Build history of the part. All positions in model axes, mm. A direction names the side the tool comes from. Give positions to 0.01 mm unless a question says otherwise; leave off trailing zeros. Loops run counter-clockwise (first coordinate to the right, second up) from the corner with the lowest first, then second, coordinate; pieces in that order, holes last. Notation, with made-up numbers: M -23,57.25 L 19,57.25 A24 cw 19,93.25 Z; hole C -29,74 d6. An arc over 180 degrees is marked long. Answer as a JSON object with one key per item and string values. Group by question number.
1. 3-axis set-ups, long thin cutter, end or side, ignore diameter. For faces 4 (the face through (18.298, -103, -40)), 5 (the face through (16.898, -103, -43)): which of +Z, -Z, +X, -X, +Y, -Y reach the whole face in a straight line?
2. Slice it at C-C (z = -36.75). List the corners of the cut face in (x, y).
3. Mould opens along Y. For faces 1 (the face through (21.729, -101.846, -48.98)), 2 (the face through (26.698, -103, -48)), 3 (the face through (21, -107.117, -47)) say: released by +Y, released by -Y, zero draft, split by the parting line, or undercut.
4. Slice it at D-D (z = -42). List the corners of the cut face in (x, y), then the cut area to 3 significant figures.
5. Drill centre lines: line 1 along Z through (x, y) = (22.5, -104.75); line 2 along Y through (x, z) = (19.75, -48.5); line 3 along Y through (x, z) = (22, -48.25). Where is each one in solid material? Low to high. Write a range as [from, to].
6. Drop flat-ended pins along their axis: pin 1 Ø1 at (x, y) = (21, -100.5) entering from +Z; pin 2 Ø3 at (y, z) = (-103.5, -36.5) entering from +X; pin 3 Ø1.4 at (y, z) = (-101.36, -48.34) entering from -X. Give the stop position or say it passes through.
7. Slice it at A-A (y = -101). List the corners of the cut face in (x, z), then the cut area to 3 significant figures.
8. Slice it at B-B (x = 26). List the corners of the cut face in (y, z).
from build123d import *

# Parameters (mm, degrees)
CROQUIS1_W                = 6
CROQUIS1_H                = 7.864261992
SALIENTE_EXTRUIR1_DEPTH   = 9.8
CROQUIS2_W                = 1.4
CROQUIS2_H                = 7.864261992
SALIENTE_EXTRUIR2_DEPTH   = 11.5
CROQUIS3_R                = 1
CORTAR_EXTRUIR1_DEPTH     = 1.4
TALADRO_ROSCADO_M21_D     = 1.6
TALADRO_ROSCADO_M21_DEPTH = 13
TALADRO_ROSCADO_M21_TIP   = 0.480688495


with BuildPart() as part:
    # Croquis1 → Saliente-Extruir1 (new body)
    with BuildSketch(Plane.ZY.offset(-26.697955236)):
        with Locations((-48.344788292, -103.185244075)):
            Rectangle(CROQUIS1_W, CROQUIS1_H)
    extrude(amount=SALIENTE_EXTRUIR1_DEPTH)

    # Croquis2 → Saliente-Extruir2 (add)
    with BuildSketch(Plane.XY.offset(-45.344788292)):
        with Locations((17.597955236, -103.185244075)):
            Rectangle(CROQUIS2_W, CROQUIS2_H)
    extrude(amount=SALIENTE_EXTRUIR2_DEPTH)

    # Croquis3 → Cortar-Extruir1 (cut)
    with BuildSketch(Plane(origin=(18.297955236, 0, 0), x_dir=(0, 0, -1), z_dir=(1, 0, 0))):
        with Locations((36.344788292, -103.185244075)):
            Circle(CROQUIS3_R)
    extrude(amount=-CORTAR_EXTRUIR1_DEPTH, mode=Mode.SUBTRACT)

    # Taladro roscado M21
    with Locations(Plane(origin=(26.697955236, 0, 0), x_dir=(0, 0, -1), z_dir=(1, 0, 0))):
        with Locations((48.344788292, -104.677829932), (48.344788292, -101.359309211)):
            Hole(TALADRO_ROSCADO_M21_D / 2, depth=TALADRO_ROSCADO_M21_DEPTH)
            with Locations((0, 0, -(TALADRO_ROSCADO_M21_DEPTH + TALADRO_ROSCADO_M21_TIP / 2))):  # 118° drill point
                Cone(0, TALADRO_ROSCADO_M21_D / 2, TALADRO_ROSCADO_M21_TIP, mode=Mode.SUBTRACT)


solid = part.part
Established:
{
 "1": {"face 4": "+Z, +X, +Y, -Y", "face 5": "+Z, -Z, -X, +Y, -Y"},
 "2": {"outline": "M 16.9,-107.12 L 18.3,-107.12 L 18.3,-104.1 L 16.9,-104.1 Z; M 16.9,-102.27 L 18.3,-102.27 L 18.3,-99.25 L 16.9,-99.25 Z"},
 "3": {"face 1": "undercut", "face 2": "zero draft", "face 3": "released by -Y"},
 "4": {"outline": "M 16.9,-107.12 L 18.3,-107.12 L 18.3,-99.25 L 16.9,-99.25 Z", "area": "11.0 mm^2"},
 "5": {"line 1": "z = [-51.34, -49.14], [-47.55, -45.34]", "line 2": "y = [-107.12, -105.46], [-103.89, -102.14], [-100.57, -99.25]", "line 3": "y = [-107.12, -105.47], [-103.88, -102.15], [-100.56, -99.25]"},
 "6": {"pin 1": "stops at z = -45.34", "pin 2": "stops at x = 18.3", "pin 3": "passes through"},
 "7": {"outline": "M 16.9,-51.34 L 26.7,-51.34 L 26.7,-49.06 L 16.9,-49.06 Z; M 16.9,-47.63 L 26.7,-47.63 L 26.7,-45.34 L 18.3,-45.34 L 18.3,-33.84 L 16.9,-33.84 Z", "area": "60.9 mm^2"},
 "8": {"outline": "M -107.12,-51.34 L -99.25,-51.34 L -99.25,-45.34 L -107.12,-45.34 Z; hole C -104.68,-48.34 d1.6; hole C -101.36,-48.34 d1.6"}
}
